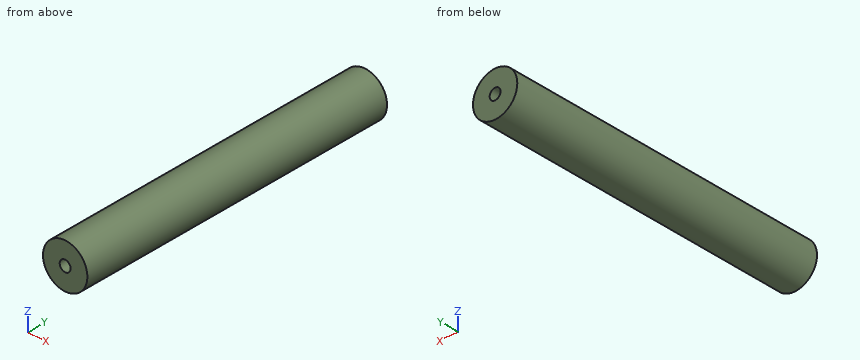
Autodesk Inventor part; units mm, degrees
ref_plane "YZ Plane" through (0, 0, 0) normal (1, 0, 0) x (0, 1, 0)
ref_plane "XZ Plane" through (0, 0, 0) normal (0, 1, 0) x (-1, 0, 0)
ref_plane "XY Plane" through (0, 0, 0) normal (0, 0, 1) x (1, 0, 0)
sketch "Sketch1" plane through (0, 0, 0) normal (0, 1, 0) x (-1, 0, 0)
  circle A0 centre (0, 0) radius 10
  dimension "d0" = 20
extrude "Extrusion1" add sketch "Sketch1" along normal blind 146.05
sketch "Sketch2" plane through (0, 146.05, 0) normal (0, 1, 0) x (1, 0, 0)
  circle A0 centre (0, 0) radius 10
  circle A1 centre (0, 0) radius 1.7528
hole "Hole1" at (0, 146.05, 0) direction (0, -1, 0) diameter 4.9276 depth 25 tip angle 118
sketch "Sketch3" plane through (0, 0, 0) normal (0, -1, 0) x (1, 0, 0)
  circle A0 centre (0, 0) radius 10
  circle A1 centre (0, 0) radius 2.7242
hole "Hole2" at (0, 0, 0) direction (0, 1, 0) diameter 4.9276 depth 25 tip angle 118
properties part number "dipoleDiscSpacer_B" material "Acetal Resin, White"
Input: part model. Units: mm. Frame: model coordinates. Round coordinates to 2 decimals unless told otherwise and drop trailing zeros. Order: outer loops, then holes, each group sorted by start corner. A loop starts at its lowest first (then second) coordinate and runs counter-clockwise, first axis right, second up. Notation, with made-up numbers: (24.25, 24) - (79.25, 24) arc R19 cw to (79.25, 58) - close; hole circle Ø3 at (-13.75, 83.5). An arc over 180 degrees is marked (long way). One line per question, with ' | ' between items. Start each with the question number.
1) Cut plane D-D, the plane z = 8.25. Return the cut outline in (x, y).
2) Ray query, probe 1 along Z at (x, y) = (0, 13.25); probe 2 along X at (y, z) = (103, 4.75); probe 3 along X at (y, z) = (31, -0.5). Return the intervals inside material, ascending.
3) Contact query for flat-ended pins moving along their axis: P1, Ø3, axis at x = -6, y = 121.5, coming from the +Z side; P2, Ø1.5, axis at x = 7.5, z = -2, coming from the -Y side; P3, Ø2, axis at x = 3, y = 91, coming from the +Z side. Output: stop coordinate, or through.
4) Cut plane B-B, the plane y = 87. Return the cut outline in (x, z), then the cut area to 3 significant figures.
5) Cut plane C-C, the plane x = -8. Return the cut outline in (y, z), then the cut area to 3 significant figures.
6) Cut plane A-A, the plane y = 129. Return the cut outline in (x, z), then the cut area to 3 significant figures.
Worked out:
1) outline: (-5.65, 0) - (5.65, 0) - (5.65, 146.05) - (-5.65, 146.05) - close
2) probe 1: z = -10 to -2.46, 2.46 to 10 | probe 2: x = -8.8 to 8.8 | probe 3: x = -9.99 to 9.99
3) P1: stops at z = 8.93 | P2: stops at y = 0 | P3: stops at z = 9.8
4) outline: circle Ø20 at (0, 0) | area: 314 mm^2
5) outline: (0, -6) - (146.05, -6) - (146.05, 6) - (0, 6) - close | area: 1,750 mm^2
6) outline: circle Ø20 at (0, 0); hole circle Ø4.93 at (0, 0) | area: 295 mm^2
